Source: CAD feature listing. Evaluate the final solid. Frame: model axes, mm. Coordinates: 2 decimals unless noted, no trailing zeros. Order: outer loops, then holes, each group sorted by start corner. A loop starts at its lowest first (then second) coordinate and runs counter-clockwise, first axis right, second up. Notation, with made-up numbers: (48.5, 89.25) -> (80.5, 89.25) arc R23 cw to (80.5, 109.25) -> close; hole circle Ø3 at (89.25, 60.5). An arc over 180 degrees is marked (long way). Write item = value, one per line. Start each with the question number.
Item 1: Section query A-A (y = 0). Output: boundary loops of the cut face in (x, z), then the cut area to 4 significant figures.
Item 2: Mould query, pull axis X, two halves, no side actions, for faces 1 (the cylindrical face through (-8.913, -10.413, 2.465)), 2 (the cylindrical face through (6.92, -9.69, 2.46)), 3 (the cylindrical face through (62, 19.52, 2.46)). Classes: released by +X, released by -X, zero draft, split by the parting line, or undercut.
Item 3: Contact query for flat-ended pins moving along their axis: pin 1 (1 mm diameter, centred on x = -48, z = 1.5, fed in from +Y); pin 2 (1.5 mm diameter, centred on x = 10, z = 1.5, fed in from -Y); pin 3 (1.5 mm diameter, centred on x = 5.5, z = 4, fed in from +Y). Output: stop coordinate, or through.
Item 4: Ray query, line 1 along X through (y, z) = (-26, 1.6); line 2 along X through (y, z) = (-54, 4.3); line 3 along X through (y, z) = (31.5, 3.25). Return the intervals inside material, ascending. Write a range as [from, to].
Item 5: Section query D-D (y = 29.25). Output: boundary loops of the cut face in (x, z).
Item 6: Section query B-B (x = 30). Output: boundary loops of the cut face in (y, z).
Item 7: Section query C-C (x = 50). Output: boundary loops of the cut face in (y, z) (3 decimals), then the cut area to 3 significant figures.
```python
from build123d import *

# Parameters (mm, degrees)
SKETCH1_R           = 65
SKETCH1_R_2         = 3.95
SKETCH1_R_3         = 2.4
SKETCH1_R_4         = 4
SKETCH1_R_5         = 1.475
SKETCH1_R_6         = 1.975
SKETCH1_W           = 13.4
SKETCH1_H           = 5
BOSS_EXTRUDE1_DEPTH = 5


with BuildPart() as part:
    # Sketch1 → Boss-Extrude1 (new body)
    with BuildSketch(Plane.XY):
        Circle(SKETCH1_R)
        Circle(SKETCH1_R_2, mode=Mode.SUBTRACT)
        with Locations((0, 52)):
            Circle(SKETCH1_R_3, mode=Mode.SUBTRACT)
        with Locations((-30, 0)):
            Circle(SKETCH1_R_3, mode=Mode.SUBTRACT)
        with Locations(Location((0, -52, 0), (0, 0, 180))):
            Circle(SKETCH1_R_3, mode=Mode.SUBTRACT)
        with Locations(Location((30, 0, 0), (0, 0, 180))):
            Circle(SKETCH1_R_3, mode=Mode.SUBTRACT)
        with Locations((-41.365746699, 41.365746699)):
            Circle(SKETCH1_R_4, mode=Mode.SUBTRACT)
        with Locations((-29.25, 50.662486121)):
            Circle(SKETCH1_R_4, mode=Mode.SUBTRACT)
        with Locations((-50.662486121, 29.25)):
            Circle(SKETCH1_R_4, mode=Mode.SUBTRACT)
        with Locations(Location((50.662486121, 29.25, 0), (0, 0, 180))):
            Circle(SKETCH1_R_4, mode=Mode.SUBTRACT)
        with Locations(Location((41.365746699, 41.365746699, 0), (0, 0, 180))):
            Circle(SKETCH1_R_4, mode=Mode.SUBTRACT)
        with Locations(Location((29.25, 50.662486121, 0), (0, 0, 180))):
            Circle(SKETCH1_R_4, mode=Mode.SUBTRACT)
        with Locations((50.662486121, -29.25)):
            Circle(SKETCH1_R_4, mode=Mode.SUBTRACT)
        with Locations((41.365746699, -41.365746699)):
            Circle(SKETCH1_R_4, mode=Mode.SUBTRACT)
        with Locations((29.25, -50.662486121)):
            Circle(SKETCH1_R_4, mode=Mode.SUBTRACT)
        with Locations(Location((-29.25, -50.662486121, 0), (0, 0, 180))):
            Circle(SKETCH1_R_4, mode=Mode.SUBTRACT)
        with Locations(Location((-41.365746699, -41.365746699, 0), (0, 0, 180))):
            Circle(SKETCH1_R_4, mode=Mode.SUBTRACT)
        with Locations(Location((-50.662486121, -29.25, 0), (0, 0, 180))):
            Circle(SKETCH1_R_4, mode=Mode.SUBTRACT)
        with Locations((-40, 10)):
            Circle(SKETCH1_R_5, mode=Mode.SUBTRACT)
        with Locations((-50, 10)):
            Circle(SKETCH1_R_5, mode=Mode.SUBTRACT)
        with Locations(Location((-40, -10, 0), (0, 0, 180))):
            Circle(SKETCH1_R_5, mode=Mode.SUBTRACT)
        with Locations(Location((-50, -10, 0), (0, 0, 180))):
            Circle(SKETCH1_R_5, mode=Mode.SUBTRACT)
        with Locations((50, -10)):
            Circle(SKETCH1_R_5, mode=Mode.SUBTRACT)
        with Locations((40, -10)):
            Circle(SKETCH1_R_5, mode=Mode.SUBTRACT)
        with Locations(Location((40, 10, 0), (0, 0, 180))):
            Circle(SKETCH1_R_5, mode=Mode.SUBTRACT)
        with Locations(Location((50, 10, 0), (0, 0, 180))):
            Circle(SKETCH1_R_5, mode=Mode.SUBTRACT)
        with Locations((-8.485281374, 8.485281374)):
            Circle(SKETCH1_R_6, mode=Mode.SUBTRACT)
        with Locations((8.485281374, 8.485281374)):
            Circle(SKETCH1_R_6, mode=Mode.SUBTRACT)
        with Locations((8.485281374, -8.485281374)):
            Circle(SKETCH1_R_6, mode=Mode.SUBTRACT)
        with Locations((-8.485281374, -8.485281374)):
            Circle(SKETCH1_R_6, mode=Mode.SUBTRACT)
        with Locations((11.7, 22.5)):
            Rectangle(SKETCH1_W, SKETCH1_H, mode=Mode.SUBTRACT)
        with Locations((-11.3, 22.5)):
            Rectangle(SKETCH1_W, SKETCH1_H, mode=Mode.SUBTRACT)
        with Locations((11.7, -22.5)):
            Rectangle(SKETCH1_W, SKETCH1_H, mode=Mode.SUBTRACT)
        with Locations((-11.3, -22.5)):
            Rectangle(SKETCH1_W, SKETCH1_H, mode=Mode.SUBTRACT)
    extrude(amount=BOSS_EXTRUDE1_DEPTH)


solid = part.part
```
Computed:
q1.outline = (-65, 0) -> (-32.4, 0) -> (-32.4, 5) -> (-65, 5) -> close; (-27.6, 0) -> (-3.95, 0) -> (-3.95, 5) -> (-27.6, 5) -> close; (3.95, 0) -> (27.6, 0) -> (27.6, 5) -> (3.95, 5) -> close; (32.4, 0) -> (65, 0) -> (65, 5) -> (32.4, 5) -> close
q1.area = 562.5 mm^2
q2.face_1 = undercut
q2.face_2 = undercut
q2.face_3 = split by the parting line
q3.pin_1 = 44.37
q3.pin_2 = -64.34
q3.pin_3 = 64.83
q4.line_1 = [-59.57, -52.99], [-48.33, 48.33], [52.99, 59.57]
q4.line_2 = [-36.18, -31.45], [-27.05, -1.33], [1.33, 27.05], [31.45, 36.18]
q4.line_3 = [-56.86, -53.97], [-47.36, 47.36], [53.97, 56.86]
q5.outline = (-58.05, 0) -> (-54.66, 0) -> (-54.66, 5) -> (-58.05, 5) -> close; (-46.66, 0) -> (46.66, 0) -> (46.66, 5) -> (-46.66, 5) -> close; (54.66, 0) -> (58.05, 0) -> (58.05, 5) -> (54.66, 5) -> close
q6.outline = (-57.66, 0) -> (-54.59, 0) -> (-54.59, 5) -> (-57.66, 5) -> close; (-46.73, 0) -> (-2.4, 0) -> (-2.4, 5) -> (-46.73, 5) -> close; (2.4, 0) -> (46.73, 0) -> (46.73, 5) -> (2.4, 5) -> close; (54.59, 0) -> (57.66, 0) -> (57.66, 5) -> (54.59, 5) -> close
q7.outline = (-41.533, 0) -> (-33.195, 0) -> (-33.195, 5) -> (-41.533, 5) -> close; (-25.305, 0) -> (-11.475, 0) -> (-11.475, 5) -> (-25.305, 5) -> close; (-8.525, 0) -> (8.525, 0) -> (8.525, 5) -> (-8.525, 5) -> close; (11.475, 0) -> (25.305, 0) -> (25.305, 5) -> (11.475, 5) -> close; (33.195, 0) -> (41.533, 0) -> (41.533, 5) -> (33.195, 5) -> close
q7.area = 307 mm^2
